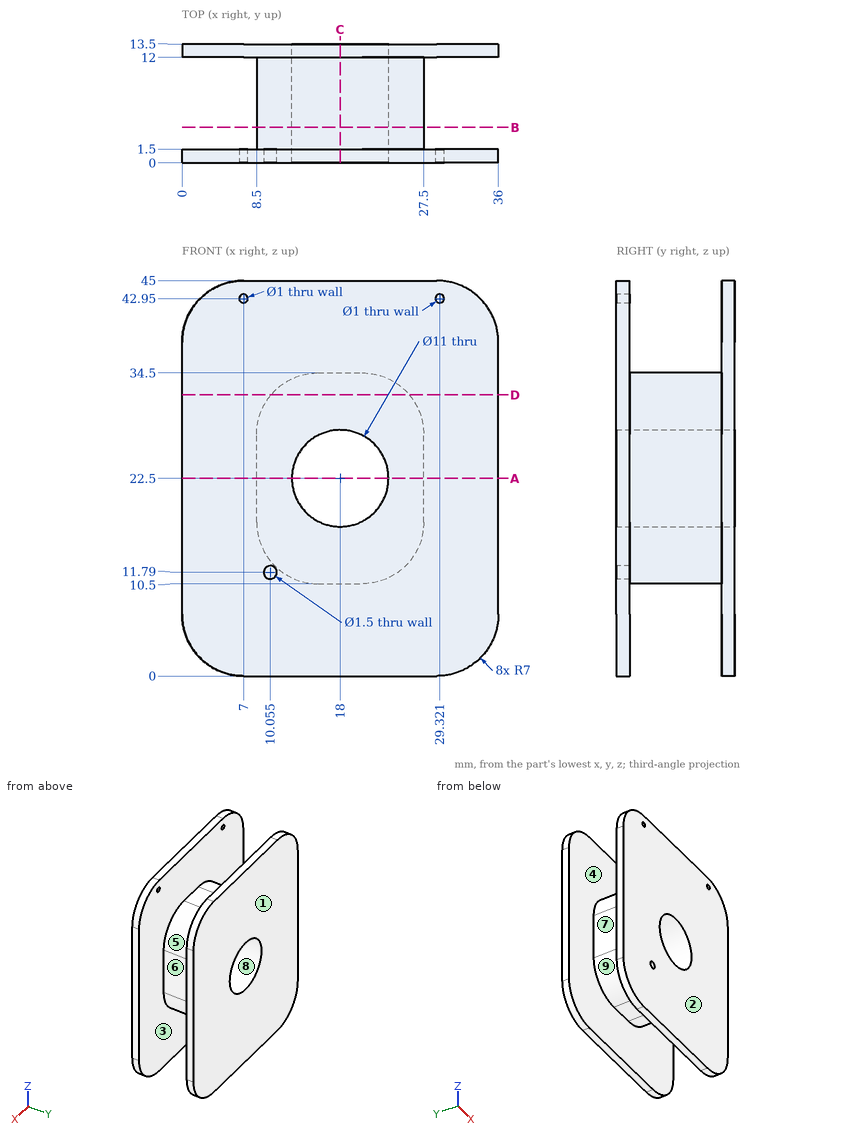
Study the drawing (mm; zero at the part's minimum x, y, z) and answer. A direction names the side the tool comes from. Round coordinates to 2 decimals unless told otherwise and drop trailing zeros. Order: outer loops, then holes, each group sorted by start corner. A loop starts at its lowest first (then second) coordinate and runs counter-clockwise, first axis right, second up. Notation, with made-up numbers: M 67.5,-3.75 L 86.5,-3.75 A15 ccw 86.5,20.25 Z; hole C 64,-5 d2. An arc over 180 degrees is marked long. One line per item, written item: value.
Q1. Find section D-D on z = 32. Write down the section's boundary in (x, y), then the cut area to 3 significant figures.
Derived:
outline: M 0,0 L 36,0 L 36,1.5 L 25.86,1.5 L 25.86,12 L 36,12 L 36,13.5 L 0,13.5 L 0,12 L 10.14,12 L 10.14,1.5 L 0,1.5 Z
area: 273 mm²
Q2. Determine the mould class of the marked faces 1, 2, 3 and 4 for opening direction Y: released by +Y, released by -Y, zero draft, split by the parting line, or undercut.
Derived:
face 1: released by +Y
face 2: released by -Y
face 3: undercut
face 4: undercut
Q3. Find section A-A on z = 22.5. Write down the section's boundary in (x, y), then the cut area to 3 significant figures.
Derived:
outline: M 0,0 L 12.5,0 L 12.5,13.5 L 0,13.5 L 0,12 L 8.5,12 L 8.5,1.5 L 0,1.5 Z; M 23.5,0 L 36,0 L 36,1.5 L 27.5,1.5 L 27.5,12 L 36,12 L 36,13.5 L 23.5,13.5 Z
area: 159 mm²
Q4. Flat-ended cylindrical pins translate along their axes: pin 1 (4 mm diameter, centred on x = 17.5, y = 5, fed in from +Z); pin 2 (6.5 mm diameter, centred on x = 18, z = 22.5, fed in from +Y); pin 3 (1.5 mm diameter, centred on x = 19, y = 5.5, fed in from -Z); pin 4 (5 mm diameter, centred on y = 6, z = 22, fed in from -X). Find the tip coordinate at first contact, or state that the pin passes through.
Derived:
pin 1: z = 34.5
pin 2: through
pin 3: z = 10.5
pin 4: x = 8.5
Q5. Straight lines are drawn through the part: line 1 (Z direction, x = 18, y = 3.5); line 2 (Y direction, x = 29, z = 11); line 3 (Z direction, x = 7, y = 0.45). For each, find the intervals that lie inside material, in ascending order.
Derived:
line 1: 10.5 to 17, 28 to 34.5
line 2: 0 to 1.5, 12 to 13.5
line 3: 0 to 42.45, 43.45 to 45
Q6. Find section B-B on y = 4. Write down the section's boundary in (x, z), then the cut area to 3 significant figures.
Derived:
outline: M 8.5,17.5 A7 ccw 15.5,10.5 L 20.5,10.5 A7 ccw 27.5,17.5 L 27.5,27.5 A7 ccw 20.5,34.5 L 15.5,34.5 A7 ccw 8.5,27.5 Z; hole C 18,22.5 d11
area: 319 mm²
Q7. For the marked faces 5, 6, 7, 8 and 9, determine the directions among +Z, -Z, +X, -X, +Y, -Y from which every point of the face is accessible in a straight line to the end or side of a thin tool.
Derived:
face 5: +Z, +X
face 6: +Z, -Z, +X
face 7: +Z, -Z, -X
face 8: +Y, -Y
face 9: -Z, -X
Q8. Find section C-C on x = 18. Write down the section's boundary in (y, z).
Derived:
outline: M 0,0 L 1.5,0 L 1.5,10.5 L 12,10.5 L 12,0 L 13.5,0 L 13.5,17 L 0,17 Z; M 0,28 L 13.5,28 L 13.5,45 L 12,45 L 12,34.5 L 1.5,34.5 L 1.5,45 L 0,45 Z
